Build history of the part. All positions in model axes, mm. Face numbers are marked on the shaded views. A direction names the side the tool comes from. Give positions to 0.01 mm unless a question says otherwise; leave off trailing zeros. Loops run counter-clockwise (first coordinate to the right, second up) from the corner with the lowest first, then second, coordinate; pieces in that order, holes last. Notation, with made-up numbers: (46.25, 10.5) -> (83.25, 10.5) arc R19 ccw to (83.25, 26.5) -> close; hole circle Ø5 at (63, -26.5). An arc over 180 degrees is marked (long way). Answer as a JSON object with one key per item and string values. Group by question number.
Q1. Drop flat-ended pins along their axis: pin 1 (6 mm diameter, centred on x = -11, z = 2.5, fed in from +Y); pin 2 (1.5 mm diameter, centred on x = -7.5, z = -15.5, fed in from -Y); pin 3 (1 mm diameter, centred on x = 25, z = -15.5, fed in from -Y). Give the stop position or say it passes through.
Q2. Band-saw the part on C-C, the plane x = -37.5. Write the cut outline in (y, z), plus the area to 3 significant figures.
Q3. Band-saw the part on A-A, the plane z = 0. Write the cut outline in (x, y).
Q4. Wall check: probe 1 along X at (y, z) = (-6, 7); probe 2 along X at (y, z) = (5, -21); probe 3 along Z at (x, y) = (21, 15). Give the ranges that are in metal, low to high. Write a range as from..to.
Q5. Band-saw the part on B-B, the plane y = 3. Write the cut outline in (x, z).
Q6. Tool access for the marked faces 1, 2 and 3: list every direction of +Z, -Z, +X, -X, +Y, -Y with a clear straight run to the whole face (end or side of a thin tool).
Q7. Band-saw the part on D-D, the plane z = 10.5. Write the cut outline in (x, y), plus the area to 3 significant figures.
from build123d import *

# Parameters (mm, degrees)
ESQUISSE2_R        = 17.5
BOSS_EXTRU_1_DEPTH = 47
ESQUISSE3_R        = 8
BOSS_EXTRU_2_DEPTH = 20
ESQUISSE4_R        = 20.5
BOSS_EXTRU_3_DEPTH = 7
ESQUISSE5_R        = 29
BOSS_EXTRU_4_DEPTH = 7
ESQUISSE6_R        = 20
BOSS_EXTRU_5_DEPTH = 24


with BuildPart() as part:
    # Esquisse2 → Boss.-Extru.1 (new body)
    with BuildSketch(Plane(origin=(0, 0, 0), x_dir=(0, 0, -1), z_dir=(1, 0, 0))):
        Circle(ESQUISSE2_R)
    extrude(amount=-BOSS_EXTRU_1_DEPTH)

    # Esquisse3 → Boss.-Extru.2 (add)
    with BuildSketch(Plane.ZY.offset(47)):
        Circle(ESQUISSE3_R)
    extrude(amount=BOSS_EXTRU_2_DEPTH)

    # Esquisse4 → Boss.-Extru.3 (add)
    with BuildSketch(Plane(origin=(0, 0, 0), x_dir=(0, 0, -1), z_dir=(1, 0, 0))):
        Circle(ESQUISSE4_R)
    extrude(amount=BOSS_EXTRU_3_DEPTH)

    # Esquisse5 → Boss.-Extru.4 (add)
    with BuildSketch(Plane(origin=(7, 0, 0), x_dir=(0, 0, -1), z_dir=(1, 0, 0))):
        with Locations((0, 8)):
            Circle(ESQUISSE5_R)
    extrude(amount=BOSS_EXTRU_4_DEPTH)

    # Esquisse6 → Boss.-Extru.5 (add)
    with BuildSketch(Plane(origin=(14, 0, 0), x_dir=(0, 0, -1), z_dir=(1, 0, 0))):
        with Locations((0, 16)):
            Circle(ESQUISSE6_R)
    extrude(amount=BOSS_EXTRU_5_DEPTH)


solid = part.part
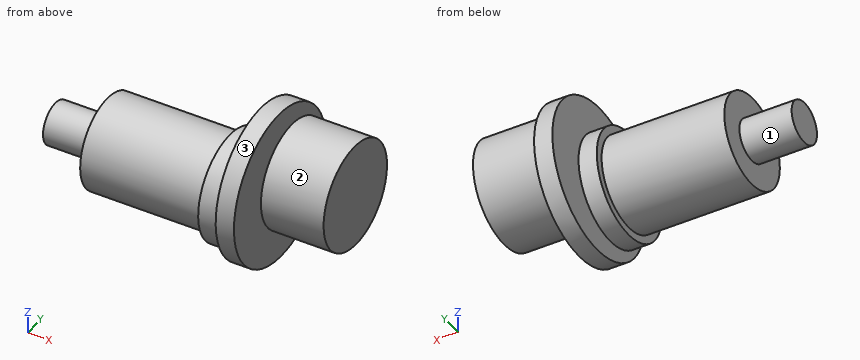
Worked answers:
{
 "1": {"pin 1": "y = 17.5", "pin 2": "y = -9.42", "pin 3": "y = 2.77"},
 "2": {"outline": "circle Ø35 at (0, 0)", "area": "962 mm2"},
 "3": {"outline": "(-67, -8) -> (-47, -8) -> (-47, -17.5) -> (0, -17.5) -> (0, -20.5) -> (7, -20.5) -> (7, -21) -> (14, -21) -> (14, -4) -> (38, -4) -> (38, 36) -> (14, 36) -> (14, 37) -> (7, 37) -> (7, 20.5) -> (0, 20.5) -> (0, 17.5) -> (-47, 17.5) -> (-47, 8) -> (-67, 8) -> close"},
 "4": {"probe 1": "-47..14", "probe 2": "7..14", "probe 3": "-19.97..19.97"},
 "5": {"outline": "(-67, -7.42) -> (-47, -7.42) -> (-47, -17.24) -> (0, -17.24) -> (0, -20.28) -> (7, -20.28) -> (7, -28.57) -> (14, -28.57) -> (14, -15.2) -> (38, -15.2) -> (38, 15.2) -> (14, 15.2) -> (14, 28.57) -> (7, 28.57) -> (7, 20.28) -> (0, 20.28) -> (0, 17.24) -> (-47, 17.24) -> (-47, 7.42) -> (-67, 7.42) -> close"},
 "6": {"face 1": "-X", "face 2": "+X", "face 3": "+X, -X"},
 "7": {"outline": "(-47, -14) -> (0, -14) -> (0, -17.61) -> (7, -17.61) -> (7, -19.03) -> (14, -19.03) -> (14, -1.02) -> (38, -1.02) -> (38, 33.02) -> (14, 33.02) -> (14, 35.03) -> (7, 35.03) -> (7, 17.61) -> (0, 17.61) -> (0, 14) -> (-47, 14) -> close", "area": "2,760 mm2"}
}
